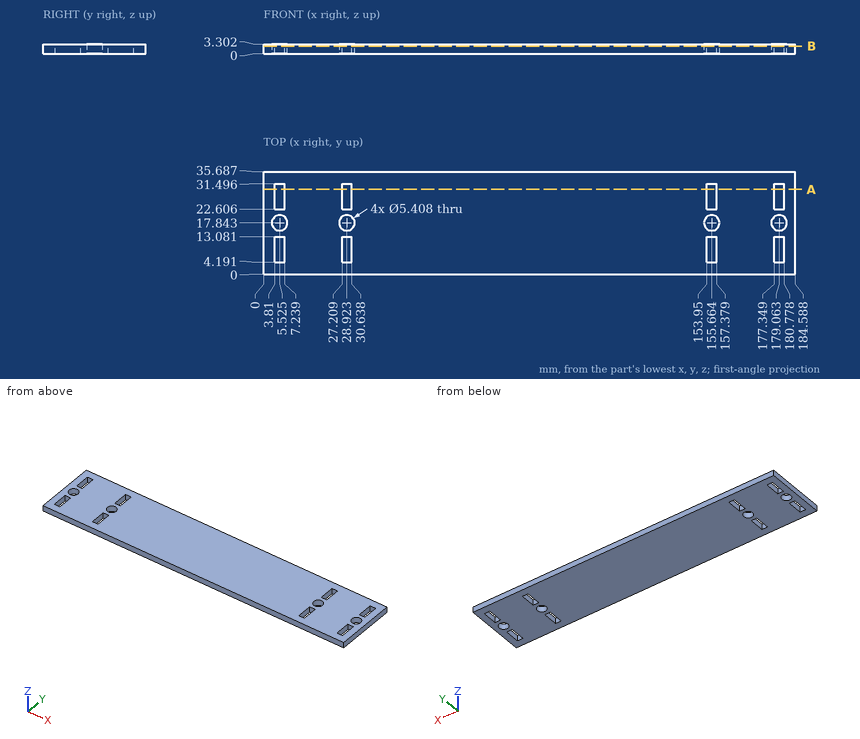
Print and shaded views of the part. All mm, measured from the part's lowest x, y and z. Give positions to 0.01 mm unless a question says otherwise; leave off trailing zeros. Order: outer loops, then holes, each group sorted by start corner. A loop starts at its lowest first (then second) coordinate and runs counter-clockwise, first axis right, second up. Notation, with made-up numbers: M -26,-32 L 20,-32 A18 ccw 20,-3 Z; hole C 1,37 d7. An arc over 180 degrees is marked long. Use one line per item in the form item = value.
Q1. Slice it at A-A, the plane y = 29.5. Write the cut outline in (x, z).
Conclusion:
outline = M 0,0 L 3.81,0 L 3.81,3.3 L 0,3.3 Z; M 7.24,0 L 27.21,0 L 27.21,3.3 L 7.24,3.3 Z; M 30.64,0 L 153.95,0 L 153.95,3.3 L 30.64,3.3 Z; M 157.38,0 L 177.35,0 L 177.35,3.3 L 157.38,3.3 Z; M 180.78,0 L 184.59,0 L 184.59,3.3 L 180.78,3.3 Z
Q2. Wall check: probe 1 along X at (y, z) = (8, 0.8); probe 2 along X at (y, z) = (18, 1.5) (1 decimal). Give the ranges that are in metal, low to high.
Conclusion:
probe_1 = 0 to 3.81, 7.24 to 27.21, 30.64 to 153.95, 157.38 to 177.35, 180.78 to 184.59
probe_2 = 0 to 2.8, 8.2 to 26.2, 31.6 to 153, 158.4 to 176.4, 181.8 to 184.6
Q3. Slice it at B-B, the plane z = 2.55. State how many separate pieces and enclosed holes the cut face has, and give its area (3 significant figures).
Conclusion:
separate_pieces = 1
enclosed_holes = 12
area = 6,250 mm2
